The figure shows three views and two pictorial views of one solid part (mm, origin at its lowest corner). Answer the questions. Give positions to 0.01 mm unless a question says otherwise; leave off trailing zeros. Loops run counter-clockwise (first coordinate to the right, second up) from the corner with the lowest first, then second, coordinate; pieces in that order, holes last. Notation, with made-up numbers: (53.5, -17.5) - (85.5, -17.5) arc R20 cw to (85.5, 7.5) - close; hole circle Ø10 at (4.25, 81.25). An arc over 180 degrees is marked (long way). One line per question, with ' | ' between items.
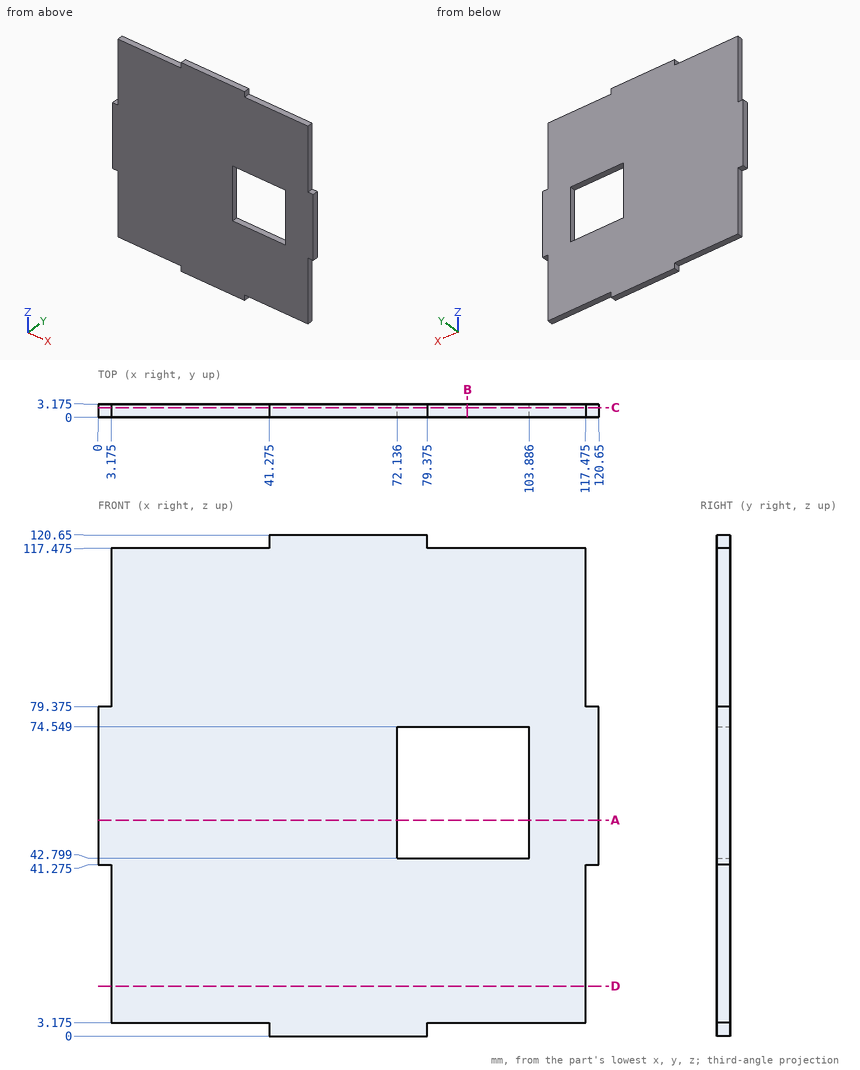
1. Find section C-C on y = 2.3. Write down the section's boundary in (x, z) (3 decimals), then the cut area to 3 significant figures.
Evaluation:
outline: (0, 41.275) - (3.175, 41.275) - (3.175, 3.175) - (41.275, 3.175) - (41.275, 0) - (79.375, 0) - (79.375, 3.175) - (117.475, 3.175) - (117.475, 41.275) - (120.65, 41.275) - (120.65, 79.375) - (117.475, 79.375) - (117.475, 117.475) - (79.375, 117.475) - (79.375, 120.65) - (41.275, 120.65) - (41.275, 117.475) - (3.175, 117.475) - (3.175, 79.375) - (0, 79.375) - close; hole (72.136, 42.799) - (103.886, 42.799) - (103.886, 74.549) - (72.136, 74.549) - close | area: 12,500 mm2
2. Find section A-A on z = 52. Write down the section's boundary in (x, y) (3 decimals), then the cut area to 3 significant figures.
Evaluation:
outline: (0, 0) - (72.136, 0) - (72.136, 3.175) - (0, 3.175) - close; (103.886, 0) - (120.65, 0) - (120.65, 3.175) - (103.886, 3.175) - close | area: 282 mm2
3. Find section B-B on x = 89. Write down the section's boundary in (y, z) (3 decimals), then the cut area to 3 significant figures.
Evaluation:
outline: (0, 3.175) - (3.175, 3.175) - (3.175, 42.799) - (0, 42.799) - close; (0, 74.549) - (3.175, 74.549) - (3.175, 117.475) - (0, 117.475) - close | area: 262 mm2
4. Flat-ended cylindrical pins translate along their axes: pin 1 (1.6 mm diameter, centred on y = 2.5, z = 1, fed in from -X) (3 decimals); pin 2 (1 mm diameter, centred on x = 95.5, y = 1.5, fed in from -Z) (3 decimals); pin 3 (1 mm diameter, centred on x = 119.5, y = 2, fed in from -Z) (3 decimals); pin 4 (6 mm diameter, centred on x = 77, z = 55, fed in from +Y). Find the tip coordinate at first contact, or state that the pin passes through.
Evaluation:
pin 1: x = 41.275 | pin 2: z = 3.175 | pin 3: z = 41.275 | pin 4: through
5. Consider L1, parallel to X at y = 2, z = 54.5; L2, parallel to Z at x = 92.5, y = 2.25 (3 decimals); L3, parallel to Z at x = 25.5, y = 1.1 (3 decimals). Determine where each line is inside the solid, lowest interval first.
Evaluation:
L1: 0 to 72.14, 103.89 to 120.65 | L2: 3.175 to 42.799, 74.549 to 117.475 | L3: 3.175 to 117.475
6. Find section D-D on z = 12. Write down the section's boundary in (x, y) (3 decimals).
Evaluation:
outline: (3.175, 0) - (117.475, 0) - (117.475, 3.175) - (3.175, 3.175) - close
